Model file for the job. Use its own axes, mm. A direction names the side the tool comes from. Coordinates: 2 decimals unless noted, no trailing zeros. Loops run counter-clockwise (first coordinate to the right, second up) from the corner with the lowest first, then second, coordinate; pieces in that order, holes last.
from build123d import *

# Parameters (mm, degrees)
ESQUISSE1_W             = 40
ESQUISSE1_H             = 40
ESQUISSE1_R             = 2
BOSS_EXTRU_1_DEPTH      = 10
ESQUISSE1_3_R           = 2
ESQUISSE1_3_R_2         = 1.25
BOSS_EXTRU_2_DEPTH      = 8
ENL_V_MAT_EXTRU_1_REACH = 59.446
ESQUISSE2_R             = 1.15
ESQUISSE2_5_R           = 3
ESQUISSE2_5_R_2         = 1.15
ENL_V_MAT_EXTRU_2_DEPTH = 4
CONG_1_SIZE             = 10


with BuildPart() as part:
    # Esquisse1 → Boss.-Extru.1 (new body)
    with BuildSketch(Plane.XY):
        with Locations((20, 20)):
            Rectangle(ESQUISSE1_W, ESQUISSE1_H)
        with Locations((20, 20)):
            Circle(ESQUISSE1_R, mode=Mode.SUBTRACT)
    extrude(amount=BOSS_EXTRU_1_DEPTH)

    # Esquisse1<3> → Boss.-Extru.2 (add)
    with BuildSketch(Plane.XY):
        with Locations((20, 20)):
            Circle(ESQUISSE1_3_R)
        with Locations((20, 20)):
            Circle(ESQUISSE1_3_R_2, mode=Mode.SUBTRACT)
    extrude(amount=BOSS_EXTRU_2_DEPTH)

    # Esquisse2 → Enlèv. mat.-Extru.1 (cut, up to next)
    with BuildSketch(Plane(origin=(0, 0, 0), x_dir=(-1, 0, 0), z_dir=(0, 0, -1)), mode=Mode.PRIVATE) as enl_v_mat_extru_1_sk1:
        with Locations((-9.039844892, 30.960155108)):
            Circle(ESQUISSE2_R)
    enl_v_mat_extru_1_tool1 = extrude(enl_v_mat_extru_1_sk1.sketch, amount=-ENL_V_MAT_EXTRU_1_REACH, mode=Mode.PRIVATE) & part.part
    # Esquisse2 → Enlèv. mat.-Extru.1 (cut, up to next)
    with BuildSketch(Plane(origin=(0, 0, 0), x_dir=(-1, 0, 0), z_dir=(0, 0, -1)), mode=Mode.PRIVATE) as enl_v_mat_extru_1_sk2:
        with Locations((-9.039844892, 9.039844892)):
            Circle(ESQUISSE2_R)
    enl_v_mat_extru_1_tool2 = extrude(enl_v_mat_extru_1_sk2.sketch, amount=-ENL_V_MAT_EXTRU_1_REACH, mode=Mode.PRIVATE) & part.part
    # Esquisse2 → Enlèv. mat.-Extru.1 (cut, up to next)
    with BuildSketch(Plane(origin=(0, 0, 0), x_dir=(-1, 0, 0), z_dir=(0, 0, -1)), mode=Mode.PRIVATE) as enl_v_mat_extru_1_sk3:
        with Locations((-30.960155108, 9.039844892)):
            Circle(ESQUISSE2_R)
    enl_v_mat_extru_1_tool3 = extrude(enl_v_mat_extru_1_sk3.sketch, amount=-ENL_V_MAT_EXTRU_1_REACH, mode=Mode.PRIVATE) & part.part
    # Esquisse2 → Enlèv. mat.-Extru.1 (cut, up to next)
    with BuildSketch(Plane(origin=(0, 0, 0), x_dir=(-1, 0, 0), z_dir=(0, 0, -1)), mode=Mode.PRIVATE) as enl_v_mat_extru_1_sk4:
        with Locations((-30.960155108, 30.960155108)):
            Circle(ESQUISSE2_R)
    enl_v_mat_extru_1_tool4 = extrude(enl_v_mat_extru_1_sk4.sketch, amount=-ENL_V_MAT_EXTRU_1_REACH, mode=Mode.PRIVATE) & part.part
    add(enl_v_mat_extru_1_tool1.solids().sort_by_distance((9.039845, 30.960155, 0))[0], mode=Mode.SUBTRACT)
    add(enl_v_mat_extru_1_tool2.solids().sort_by_distance((9.039845, 9.039845, 0))[0], mode=Mode.SUBTRACT)
    add(enl_v_mat_extru_1_tool3.solids().sort_by_distance((30.960155, 9.039845, 0))[0], mode=Mode.SUBTRACT)
    add(enl_v_mat_extru_1_tool4.solids().sort_by_distance((30.960155, 30.960155, 0))[0], mode=Mode.SUBTRACT)

    # Esquisse2<5> → Enlèv. mat.-Extru.2 (cut)
    # profile 1 of 4: a face of its own
    with BuildSketch(Plane(origin=(0, 0, 0), x_dir=(-1, 0, 0), z_dir=(0, 0, -1))):
        with Locations((-9.039844892, 30.960155108)):
            Circle(ESQUISSE2_5_R)
        with Locations((-9.039844892, 30.960155108)):
            Circle(ESQUISSE2_5_R_2, mode=Mode.SUBTRACT)
    # profile 2 of 4: a face of its own
    with BuildSketch(Plane(origin=(0, 0, 0), x_dir=(-1, 0, 0), z_dir=(0, 0, -1))):
        with Locations((-9.039844892, 9.039844892)):
            Circle(ESQUISSE2_5_R)
        with Locations((-9.039844892, 9.039844892)):
            Circle(ESQUISSE2_5_R_2, mode=Mode.SUBTRACT)
    # profile 3 of 4: a face of its own
    with BuildSketch(Plane(origin=(0, 0, 0), x_dir=(-1, 0, 0), z_dir=(0, 0, -1))):
        with Locations((-30.960155108, 9.039844892)):
            Circle(ESQUISSE2_5_R)
        with Locations((-30.960155108, 9.039844892)):
            Circle(ESQUISSE2_5_R_2, mode=Mode.SUBTRACT)
    # profile 4 of 4: a face of its own
    with BuildSketch(Plane(origin=(0, 0, 0), x_dir=(-1, 0, 0), z_dir=(0, 0, -1))):
        with Locations((-30.960155108, 30.960155108)):
            Circle(ESQUISSE2_5_R)
        with Locations((-30.960155108, 30.960155108)):
            Circle(ESQUISSE2_5_R_2, mode=Mode.SUBTRACT)
    extrude(amount=-ENL_V_MAT_EXTRU_2_DEPTH, mode=Mode.SUBTRACT)

    # Congé1
    # a fillet whose section is not a circle: 10 mm, written as the material it takes off along each edge
    with BuildSketch(Plane(origin=(0, 0, -25), x_dir=(1, 0, 0), z_dir=(0, 0, 1)), Plane(origin=(0, 40, -25), x_dir=(0, -1, 0), z_dir=(0, 0, 1))) as cong_1_piece_1:
        with BuildLine():
            add(Edge.make_bspline([(CONG_1_SIZE, 0), (CONG_1_SIZE * 0.831801948466, 0), (CONG_1_SIZE * 0.663603896932, 0), (CONG_1_SIZE * 0.292893218813, CONG_1_SIZE * 0.0716919198361), (CONG_1_SIZE * 0.0716919198361, CONG_1_SIZE * 0.292893218813), (0, CONG_1_SIZE * 0.663603896932), (0, CONG_1_SIZE * 0.831801948466), (0, CONG_1_SIZE)], knots=[0, 0, 0, 0, 0, 0, 0.5, 0.5, 1, 1, 1, 1, 1, 1], degree=5))
            Line((0, CONG_1_SIZE), (0, 0))
            Line((0, 0), (CONG_1_SIZE, 0))
        make_face()
    extrude(amount=60, mode=Mode.SUBTRACT)
    with BuildSketch(Plane(origin=(40, 40, -25), x_dir=(0, -1, 0), z_dir=(0, 0, 1)), Plane(origin=(40, 0, -25), x_dir=(-1, 0, 0), z_dir=(0, 0, 1))) as cong_1_piece_2:
        with BuildLine():
            add(Edge.make_bspline([(CONG_1_SIZE, 0), (CONG_1_SIZE * 0.831801948466, 0), (CONG_1_SIZE * 0.663603896932, 0), (CONG_1_SIZE * 0.292893218813, -CONG_1_SIZE * 0.0716919198361), (CONG_1_SIZE * 0.0716919198361, -CONG_1_SIZE * 0.292893218813), (0, -CONG_1_SIZE * 0.663603896932), (0, -CONG_1_SIZE * 0.831801948466), (0, -CONG_1_SIZE)], knots=[0, 0, 0, 0, 0, 0, 0.5, 0.5, 1, 1, 1, 1, 1, 1], degree=5))
            Line((0, -CONG_1_SIZE), (0, 0))
            Line((0, 0), (CONG_1_SIZE, 0))
        make_face()
    extrude(amount=60, mode=Mode.SUBTRACT)


solid = part.part
Q1. Which spindle directions (+Z, -Z, +X, -X, +Y, -Y) get a long thin tool onto all of the face, cutting with end or side? Do faces 4 (the flat face through (21, 21, 8)), 5 (the cylindrical face through (31.61, 28.03, 1.97)), 6 (the cylindrical face through (30.43, 29.94, 6.96)). Say none if no direction does.
Answers:
face 4: +Z
face 5: -Z
face 6: +Z, -Z
Q2. Slice it at A-A (y = 20). List the corners of the cut face in (x, z).
Answers:
outline: (0, 0) - (18.75, 0) - (18.75, 8) - (18, 8) - (18, 10) - (0, 10) - close; (21.25, 0) - (40, 0) - (40, 10) - (22, 10) - (22, 8) - (21.25, 8) - close
Q3. Slice it at C-C (y = 31.5). Count the separate pieces of the cut face and the enclosed holes in it, and give its area (3 significant figures).
Answers:
separate pieces: 3
enclosed holes: 0
area: 328 mm2
Q4. Drill centre lines: line 1 (Y direction, x = 31, z = 5.5); line 2 (Y direction, x = 8, z = 4.5); line 3 (X direction, y = 10.5, z = 3.75). Where is each one in solid material? Low to high.
Answers:
line 1: y = 0.01 to 7.89, 10.19 to 29.81, 32.11 to 39.99
line 2: y = 0.04 to 8.55, 9.53 to 30.47, 31.45 to 39.96
line 3: x = 0 to 6.42, 11.66 to 28.34, 33.58 to 40
Q5. Mould opens along X. For faces 1 (the flat face through (7.7, 9.1, 4)), 2 (the flat face through (0, 20, 5)), 3 (the flat face through (40, 20, 5)) say: +X half, -X half, draft (parallel to the pull), parting line (faces both ways), or undercut.
Answers:
face 1: undercut
face 2: -X half
face 3: +X half
Q6. Flat gauge pins, fed straight in: P1, Ø1.2, axis at x = 19.5, y = 19, coming from the +Z side; P2, Ø1.8, axis at x = 9.5, y = 31, coming from the -Z side. Where does each tip first touch, or does it go through?
Answers:
P1: stops at z = 8
P2: stops at z = 4
